Autodesk Inventor part; units mm, degrees
ref_plane "YZ Plane" through (0, 0, 0) normal (1, 0, 0) x (0, 1, 0)
ref_plane "XZ Plane" through (0, 0, 0) normal (0, 1, 0) x (-1, 0, 0)
ref_plane "XY Plane" through (0, 0, 0) normal (0, 0, 1) x (1, 0, 0)
sketch "Sketch1" plane through (0, 0, 0) normal (0, 1, 0) x (-1, 0, 0)
  circle A0 centre (0, 0) radius 295
  dimension "d0" = 590
extrude "Extrusion1" add sketch "Sketch1" against normal blind 25
shell "Shell1" thickness 3 removed faces 1 at (-85.1519, -25, 3.4761)
fillet "Fillet1" radius 3.175 1 edges at (295, 0, 0)
properties part number "still_cover"
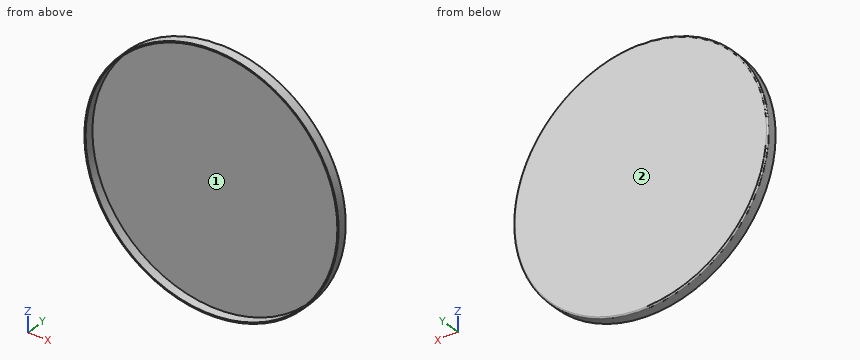
For this review, take the finished solid that the model builds, in its own axes (mm). Face numbers are marked on the shaded views. Coordinates: 2 decimals unless noted, no trailing zeros. Write each loop counter-clockwise with the first axis right and the second up, starting at its lowest first coordinate (ties: lowest second). Pieces come first, ordered by that corner, then holes.
(1) Add section B-B on z = 0. Give the boundary of the cut face in (x, y) (3 decimals).
(2) Add section C-C on y = -7.25. Give the boundary of the cut face in (x, z).
(3) Add section A-A on x = 0. Give the boundary of the cut face in (y, z) (3 decimals).
(4) Wall thickness on probe 1 along Z at (x, y) = (0, -8.5); probe 2 along Z at (x, y) = (-5, -7); probe 3 along Y at (x, z) = (23.5, 110.5): over which ranges is each line inside the solid? List them lowest first.
(5) For pin 1 Ø2 at (x, y) = (-140.5, -10) entering from +Z; pin 2 Ø10 at (y, z) = (-5, -116.5) entering from -X; pin 3 Ø10 at (y, z) = (-9, -172) entering from +X, all flat-tipped, find the tip position at first contact; note any pin that passes through.
(6) The part is to be moulded in two halves that separate along Z. For the marked faces 1 and 2, say which applies: +Z half, -Z half, draft (parallel to the pull), parting line (faces both ways), or undercut.
Answer sheet:
1. outline: (-295, -25) - (-292, -25) - (-292, -3) - (292, -3) - (292, -25) - (295, -25) - (295, -3.175) arc R3.175 ccw to (291.825, 0) - (-291.825, 0) arc R3.175 ccw to (-295, -3.175) - close
2. outline: circle Ø590 at (0, 0); hole circle Ø584 at (0, 0)
3. outline: (-25, -295) - (-3.175, -295) arc R3.175 ccw to (0, -291.825) - (0, 291.825) arc R3.175 ccw to (-3.175, 295) - (-25, 295) - (-25, 292) - (-3, 292) - (-3, -292) - (-25, -292) - close
4. probe 1: z = -295 to -292, 292 to 295
4. probe 2: z = -294.96 to -291.96, 291.96 to 294.96
4. probe 3: y = -3 to 0
5. pin 1: stops at z = 259.93
5. pin 2: stops at x = -273.12
5. pin 3: stops at x = 243.18
6. face 1: undercut
6. face 2: draft
